Source: CAD feature listing. Evaluate the final solid. Frame: model axes, mm. Face numbers are marked on the shaded views. Give positions to 0.01 mm unless a question says otherwise; leave off trailing zeros. Write item = value, one per line.
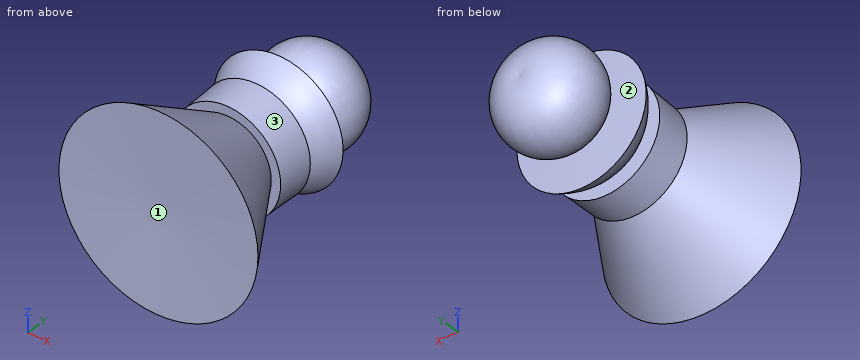
from build123d import *


with BuildPart() as f1:
    # F0 (on Top) → F1 (revolve)
    with BuildSketch(Plane.XY):
        with BuildLine():
            Line((12.6839522272, 38.5081134737), (3.8605679486, 38.5081134737))
            ThreePointArc((3.8605679486, 38.5081134737), (9.5041549163, 48.0122683899), (0, 53.6558553576))
            Line((0, 53.6558553576), (1.3687721221, 8.7601393461))
            Line((1.3687721221, 8.7601393461), (20.1665721834, 8.7601393461))
            Line((20.1665721834, 8.7601393461), (9.2163970694, 25.5504064262))
            Line((9.2163970694, 25.5504064262), (11.0414242372, 25.5504064262))
            Line((11.0414242372, 25.5504064262), (11.0414242372, 32.6680205762))
            Line((11.0414242372, 32.6680205762), (7.9928714119, 32.6680205762))
            ThreePointArc((7.9928714119, 32.6680205762), (10.7428781159, 35.2631776582), (12.6839522272, 38.5081134737))
        make_face()
    revolve(axis=Axis((0.684386061, 31.2079973519, 0), (0.030473652, -0.9995355704, 0)))


solid = f1.part
(1) Material intervals for line 1 (Y direction, x = 10, z = -3.5); line 2 (Y direction, x = -8, z = 0); line 3 (Y direction, x = -4, z = -1.5), sorted ascending.
Values follow:
line_1 = 8.74 to 23.33, 25.53 to 32.65, 35.1 to 38.49
line_2 = 8.19 to 24.14, 25.01 to 32.14, 33.14 to 37.99, 41.69 to 50.27
line_3 = 8.43 to 38.23, 38.68 to 53.28
(2) Pull-direction query (Y, two-part tool) for the marked faces 1, 2 and 3; classes: pulls with the +Y half, pulls with the -Y half, needs draft (parallel to the pull), parting line crosses it, or undercut.
Values follow:
face_1 = pulls with the -Y half
face_2 = undercut
face_3 = undercut
(3) First-contact query: pin 1 (2 mm diameter, centred on x = -5.5, z = 10, fed in from -Y); pin 2 (4 mm diameter, centred on x = 3.5, z = -5, fed in from -Y) (3 decimals); pin 3 (12 mm diameter, centred on y = 25.5, z = -9.5, fed in from +X). Flat tips, straight axial feed; report the tip coordinate or a pass-through.
Values follow:
pin_1 = 8.13
pin_2 = 8.585
pin_3 = 10.7
